```python
from build123d import *

# Parameters (mm, degrees)
F3_R     = 18.5
F4_DEPTH = 5
F5_R     = 3
F6_DEPTH = 5
F7_R     = 1.1
F8_DEPTH = 6


with BuildPart() as f2:
    # F1 (on Front) → F2 (revolve)
    with BuildSketch(Plane.XZ):
        Polygon((0, 8), (0, 0), (22.5, 0), (20, 4), (22.5, 8), align=None)
    revolve(axis=Axis((0, 0, 4), (0, 0, -1)))

    # F3 (on face) → F4 (cut)
    with BuildSketch(Plane.XY.offset(8)):
        Circle(F3_R)
    extrude(amount=-F4_DEPTH, mode=Mode.SUBTRACT)

    # F5 (on face) → F6 (join, through all)
    with BuildSketch(Plane.XY.offset(3)):
        Circle(F5_R)
    extrude(amount=F6_DEPTH)

    # F7 (on face) → F8 (cut)
    with BuildSketch(Plane.XY.offset(8)):
        Circle(F7_R)
    extrude(amount=-F8_DEPTH, mode=Mode.SUBTRACT)


solid = f2.part
```
Build history of the part. All positions in model axes, mm. A direction names the side the tool comes from. Coordinates: 2 decimals unless noted, no trailing zeros. Order: outer loops, then holes, each group sorted by start corner. A loop starts at its lowest first (then second) coordinate and runs counter-clockwise, first axis right, second up.
Item 1: Tool access for faces 4 (the conical face through (9.28, 17.85, 3.81)), 5 (the cylindrical face through (-3, 0, 5)), 6 (the flat face through (1.3, 0, 8)): list every direction of +Z, -Z, +X, -X, +Y, -Y with a clear straight run to the whole face (end or side of a thin tool).
Filled in:
face 4: none
face 5: +Z
face 6: +Z, +X, -X, +Y, -Y
Item 2: Saw through at A-A on z = 6. List the corners of the cut face in (x, y).
Filled in:
outline: circle Ø42.5 at (0, 0); circle Ø6 at (0, 0); hole circle Ø37 at (0, 0); hole circle Ø2.2 at (0, 0)
Item 3: Drop flat-ended pins along their axis: pin 1 Ø3 at (x, z) = (13.5, 3) entering from +Y; pin 2 Ø2 at (x, y) = (15, -10.5) entering from -Z; pin 3 Ø3 at (x, y) = (7.5, 14) entering from +Z. Give the stop position or say it passes through.
Filled in:
pin 1: stops at y = 17.28
pin 2: stops at z = 0
pin 3: stops at z = 3
Item 4: Saw through at B-B on y = 0. List the corners of the cut face in (x, z), then the cut area to 3 significant figures.
Filled in:
outline: (-22.5, 0) - (22.5, 0) - (20, 4) - (22.5, 8) - (18.5, 8) - (18.5, 3) - (3, 3) - (3, 8) - (1.1, 8) - (1.1, 2) - (-1.1, 2) - (-1.1, 8) - (-3, 8) - (-3, 3) - (-18.5, 3) - (-18.5, 8) - (-22.5, 8) - (-20, 4) - close
area: 172 mm2
Item 5: Drill centre lines: L1, parallel to X at y = 2, z = 7.5; L2, parallel to Y at x = 1, z = 6; L3, parallel to Y at x = 0, z = 5.1. Where is each one in solid material? Low to high.
Filled in:
L1: x = -22.1 to -18.39, -2.24 to 2.24, 18.39 to 22.1
L2: y = -21.23 to -18.47, -2.83 to -0.46, 0.46 to 2.83, 18.47 to 21.23
L3: y = -20.69 to -18.5, -3 to -1.1, 1.1 to 3, 18.5 to 20.69
Item 6: Mould opens along X. For faces 1 (the conical face through (19.226, -6.054, 4.25)), 2 (the flat face through (0, 0, 0)), 3 (the cylindrical face through (-4.01, -18.06, 5.54)) say: released by +X, released by -X, zero draft, split by the parting line, or undercut.
Filled in:
face 1: split by the parting line
face 2: zero draft
face 3: undercut
